Part model, mm, in its own coordinate system. A direction names the side the tool comes from. Give positions to 0.01 mm unless a question says otherwise; leave off trailing zeros. Write each loop counter-clockwise with the first axis right and the second up, starting at its lowest first coordinate (ties: lowest second). Pieces come first, ordered by that corner, then holes. Notation, with made-up numbers: M -17.5,-20.5 L 25.5,-20.5 A15 cw 25.5,-0.5 Z; hole C 10.5,4.25 d6. An arc over 180 degrees is marked long. Answer as CSV lines item,"result". Start each with the question number.
1) Slice it at B-B, the plane y = -23. Give the cut face in (x, z), plus the area to 3 significant figures.
2) Mould opens along Z. For faces 1 (the cylindrical face through (1.564, -18.783, -74.448)), 2 (the flat face through (1, -19, -49.044)), 3 (the cylindrical face through (2.12, -18.78, 27.16)), 4 (the flat face through (27.244, -19, -24)) say: pulls with the +Z half, pulls with the -Z half, needs draft (parallel to the pull), parting line crosses it, or undercut.
3) Slice it at C-C, the plane z = 30. Give the cut face in (x, y), plus the area to 3 significant figures.
4) Tool access for faces 5 (the flat face through (1, -19, 1.756)), 6 (the cylindrical face through (125.025, -18.783, -83.523)): list every direction of +Z, -Z, +X, -X, +Y, -Y with a clear straight run to the whole face (end or side of a thin tool).
5) Slice it at A-A, the plane z = -32. Give the cut face in (x, y).
6) Pin check, flat tips, straight feed: pin 1 Ø5 at (x, y) = (5.5, -11) entering from -Z; pin 2 Ø11.5 at (x, y) = (6.5, -14) entering from +Z. Stop position of each tip, or through.
7) Wall check: line 1 along X through (y, z) = (-7.5, -26); line 2 along Z through (x, y) = (24, -20); line 3 along X through (y, z) = (-2.5, -76.5). Give the ranges that are in metal, low to high. Write a range as from..to.
```python
from build123d import *

# Parameters (mm, degrees)
F0_W     = 50.8
F0_H     = 50.8
F1_DEPTH = 38.1


with BuildPart() as f1:
    # F0 (on Front) → F1 (new body)
    with BuildSketch(Plane.XZ):
        with BuildLine():
            Line((-10.856453, 39.855531), (-112.456453, 39.855531))
            ThreePointArc((-112.456453, 39.855531), (-121.436709, 36.135787), (-125.156453, 27.155531))
            Line((-125.156453, 27.155531), (-125.156453, -74.444469))
            ThreePointArc((-125.156453, -74.444469), (-121.436709, -83.424726), (-112.456453, -87.144469))
            Line((-112.456453, -87.144469), (-10.856453, -87.144469))
            ThreePointArc((-10.856453, -87.144469), (1.843547, -74.444469), (14.543547, -87.144469))
            Line((14.543547, -87.144469), (116.143547, -87.144469))
            ThreePointArc((116.143547, -87.144469), (125.123804, -83.424726), (128.843547, -74.444469))
            Line((128.843547, -74.444469), (128.843547, 27.155531))
            ThreePointArc((128.843547, 27.155531), (125.123804, 36.135787), (116.143547, 39.855531))
            Line((116.143547, 39.855531), (14.543547, 39.855531))
            ThreePointArc((14.543547, 39.855531), (1.843547, 27.155531), (-10.856453, 39.855531))
        make_face()
        with Locations((1.843547, -23.644469)):
            Rectangle(F0_W, F0_H, mode=Mode.SUBTRACT)
    extrude(amount=F1_DEPTH)


solid = f1.part
```
Found:
1,outline,"M -125.16,-74.44 A12.7 ccw -112.46,-87.14 L -10.86,-87.14 A12.7 cw 14.54,-87.14 L 116.14,-87.14 A12.7 ccw 128.84,-74.44 L 128.84,27.16 A12.7 ccw 116.14,39.86 L 14.54,39.86 A12.7 cw -10.86,39.86 L -112.46,39.86 A12.7 ccw -125.16,27.16 Z; hole M -23.56,-49.04 L 27.24,-49.04 L 27.24,1.76 L -23.56,1.76 Z"
1,area,"29,000 mm²"
2,face 1,"pulls with the -Z half"
2,face 2,"undercut"
2,face 3,"pulls with the +Z half"
2,face 4,"undercut"
3,outline,"M -124.83,-38.1 L -6.17,-38.1 L -6.17,0 L -124.83,0 Z; M 9.85,-38.1 L 128.52,-38.1 L 128.52,0 L 9.85,0 Z"
3,area,"9,040 mm²"
4,face 5,"+Y, -Y"
4,face 6,"-Z, +X, +Y, -Y"
5,outline,"M -125.16,-38.1 L -23.56,-38.1 L -23.56,0 L -125.16,0 Z; M 27.24,-38.1 L 128.84,-38.1 L 128.84,0 L 27.24,0 Z"
6,pin 1,"z = -76.04"
6,pin 2,"z = 32.58"
7,line 1,"-125.16..-23.56, 27.24..128.84"
7,line 2,"-87.14..-49.04, 1.76..39.86"
7,line 3,"-124.99..-5.08, 8.77..128.68"
